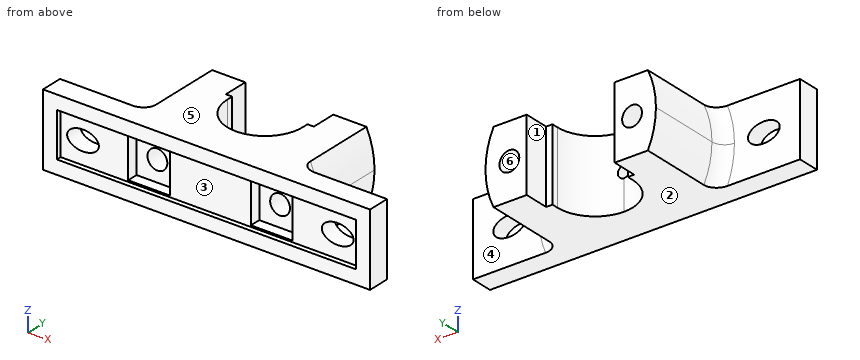
from build123d import *

# Parameters (mm, degrees)
BOSS_EXTRUDE1_DEPTH = 18.25
CUT_EXTRUDE1_START  = -43
CUT_EXTRUDE1_DEPTH  = 48
SKETCH6_R           = 5
CUT_EXTRUDE3_DEPTH  = 54.1
SKETCH7_RX          = 8
SKETCH7_RY          = 5
CUT_EXTRUDE4_DEPTH  = 11.1
FILLET3_R           = 6.4
SKETCH10_W          = 151
SKETCH10_H          = 22.5
CUT_EXTRUDE7_DEPTH  = 2.5
SKETCH11_W          = 21
SKETCH11_H          = 21
CUT_EXTRUDE8_DEPTH  = 8


with BuildPart() as part:
    # Sketch2 → Boss-Extrude1 (new, symmetric)
    with BuildSketch(Plane.XY):
        with BuildLine():
            Line((0, 0), (0, 11.1))
            Line((0, 11.1), (39.5, 11.1))
            Line((39.5, 11.1), (39.5, 54.1))
            Line((39.5, 54.1), (60.3, 54.1))
            Line((60.3, 54.1), (60.3, 41.4))
            Line((60.3, 41.4), (63.5, 41.4))
            Line((63.5, 41.4), (63.5, 38.2))
            ThreePointArc((63.5, 38.2), (69.064971157, 24.764971157), (82.5, 19.2))
            Line((82.5, 19.2), (82.5, 0))
            Line((82.5, 0), (0, 0))
        make_face()
    extrude(amount=BOSS_EXTRUDE1_DEPTH, both=True)

    # Sketch3 → Cut-Extrude1 (cut)
    with BuildSketch(Plane(origin=(0, 54.1, 0), x_dir=(1, 0, 0), z_dir=(0, 1, 0)).offset(CUT_EXTRUDE1_START)):
        with BuildLine():
            Line((39.5, -18.25), (43.564957943, -18.25))
            ThreePointArc((43.564957943, -18.25), (40.528540599, -9.348614644), (39.5, 0))
            Line((39.5, 0), (39.5, -18.25))
        make_face()
    cut_extrude1 = extrude(amount=CUT_EXTRUDE1_DEPTH, mode=Mode.SUBTRACT)

    # Mirror2: Cut-Extrude1 across plane
    add(cut_extrude1.mirror(Plane.XY), mode=Mode.SUBTRACT)

    # Mirror3: part across plane


with BuildPart() as part_1:
    add(part.part)
    add(part.part.mirror(Plane(origin=(82.5, 19.2, 18.25), x_dir=(0, 0, 1), z_dir=(1, 0, 0))))

    # Sketch6 → Cut-Extrude3 (cut)
    with BuildSketch(Plane(origin=(0, 54.1, 0), x_dir=(1, 0, 0), z_dir=(0, 1, 0))):
        with Locations(Location((51.55, 0, 0), (0, 0, 270))):
            Circle(SKETCH6_R)
    cut_extrude3 = extrude(amount=-CUT_EXTRUDE3_DEPTH, mode=Mode.SUBTRACT)

    # Sketch7 → Cut-Extrude4 (cut)
    with BuildSketch(Plane(origin=(0, 11.1, 0), x_dir=(1, 0, 0), z_dir=(0, 1, 0))):
        with Locations((18.25, 0)):
            Ellipse(SKETCH7_RX, SKETCH7_RY)
    cut_extrude4 = extrude(amount=-CUT_EXTRUDE4_DEPTH, mode=Mode.SUBTRACT)

    # Mirror4: Cut-Extrude3, Cut-Extrude4 across plane
    add(cut_extrude3.mirror(Plane.ZY.offset(-82.5)), mode=Mode.SUBTRACT)
    add(cut_extrude4.mirror(Plane.ZY.offset(-82.5)), mode=Mode.SUBTRACT)

    # Fillet3
    fillet3_edges = [part_1.edges().sort_by_distance(p)[0] for p in [
        (39.5, 11.1, 0),
        (125.5, 11.1, 0),
    ]]
    fillet(fillet3_edges, radius=FILLET3_R)

    # Sketch10 → Cut-Extrude7 (cut)
    with BuildSketch(Plane.XZ):
        with Locations((82.5, 0)):
            Rectangle(SKETCH10_W, SKETCH10_H)
    extrude(amount=-CUT_EXTRUDE7_DEPTH, mode=Mode.SUBTRACT)

    # Sketch11 → Cut-Extrude8 (cut)
    with BuildSketch(Plane.XZ):
        with Locations((51.55, 0)):
            Rectangle(SKETCH11_W, SKETCH11_H)
    cut_extrude8 = extrude(amount=-CUT_EXTRUDE8_DEPTH, mode=Mode.SUBTRACT)

    # Mirror5: Cut-Extrude8 across plane
    add(cut_extrude8.mirror(Plane.ZY.offset(-82.5)), mode=Mode.SUBTRACT)

    # Sketch12 → Cut-Revolve1 (revolve, cut)
    with BuildSketch(Plane.ZY.offset(-82.5)):
        Polygon((0, 19.5), (3, 19.5), (3, 13.5), (0, 9.983740964), align=None)
    revolve(axis=Axis((82.5, 59.1, 0), (0, -1, 0)), mode=Mode.SUBTRACT)


solid = part_1.part
CAD build for the part. Positions are in the model's coordinates, mm. Face numbers are marked on the shaded views. A direction names the side the tool comes from. Round coordinates to 2 decimals unless told otherwise and drop trailing zeros. Write each loop counter-clockwise with the first axis right and the second up, starting at its lowest first coordinate (ties: lowest second). Pieces come first, ordered by that corner, then holes.
(1) Slice it at A-A, the plane y = 47. Write the cut outline in (x, z).
(2) 3-axis set-ups, long thin cutter, end or side, ignore diameter. For the marked faces 1, 2 and 3: which of +Z, -Z, +X, -X, +Y, -Y reach the whole face in a straight line?
(3) Slice it at D-D, the plane y = 15. Write the cut outline in (x, z), and give its area (4 significant figures).
(4) Mould opens along Z. For the marked faces 4, 5 and 6 say: pulls with the +Z half, pulls with the -Z half, needs draft (parallel to the pull), parting line crosses it, or undercut.
(5) Drop flat-ended pins along their axis: P1, Ø3.5, axis at y = 39, z = 1, coming from the +X side; P2, Ø7, axis at x = 82.5, z = 0, coming from the +Y side; P3, Ø10, axis at y = 51, z = 8, coming from the +X side; P4, Ø3, axis at x = 22.5, z = -1, coming from the -Y side. Give the stop position or say it passes through.
(6) Probe line 1 along X through (y, z) = (43, 0); line 2 along Z through (x, y) = (18, 8); line 3 along X through (y, z) = (27, 0). List the from-to ranges inside material, lowest first.
(7) Slice it at B-B, the plane x = 51.55. Write the cut outline in (y, z).
(8) Slice it at C-C, the plane y = 33.5. Write the cut outline in (x, z), and give its area (3 significant figures).
From the geometry:
1. outline: (43.56, -18.25) - (60.3, -18.25) - (60.3, 18.25) - (43.56, 18.25) arc R43 ccw to start; (104.7, -18.25) - (121.44, -18.25) arc R43 ccw to (121.44, 18.25) - (104.7, 18.25) - close; hole circle Ø10 at (51.55, 0); hole circle Ø10 at (113.45, 0)
2. face 1: +Z, -Z, +Y
2. face 2: -Z, +X, -X, +Y, -Y
2. face 3: -Y
3. outline: (43, -18.25) - (122, -18.25) arc R43.51 ccw to (122, 18.25) - (43, 18.25) arc R43.51 ccw to start; hole circle Ø10 at (51.55, 0); hole circle Ø6 at (82.5, 0); hole circle Ø10 at (113.45, 0)
3. area: 2,895 mm2
4. face 4: needs draft
4. face 5: pulls with the +Z half
4. face 6: undercut
5. P1: stops at x = 125.5
5. P2: stops at y = 19.53
5. P3: stops at x = 125.4
5. P4: passes through
6. line 1: x = 39.5 to 46.55, 56.55 to 60.3, 104.7 to 108.45, 118.45 to 125.5
6. line 2: z = -18.25 to -5, 5 to 18.25
6. line 3: x = 39.5 to 46.55, 56.55 to 67.15, 97.85 to 108.45, 118.45 to 125.5
7. outline: (0, -18.25) - (54.1, -18.25) - (54.1, -5) - (8, -5) - (8, -10.5) - (2.5, -10.5) - (2.5, -11.25) - (0, -11.25) - close; (0, 11.25) - (2.5, 11.25) - (2.5, 10.5) - (8, 10.5) - (8, 5) - (54.1, 5) - (54.1, 18.25) - (0, 18.25) - close
8. outline: (43.56, -18.25) - (64.09, -18.25) - (64.09, 18.25) - (43.56, 18.25) arc R43 ccw to start; (100.91, -18.25) - (121.44, -18.25) arc R43 ccw to (121.44, 18.25) - (100.91, 18.25) - close; hole circle Ø10 at (51.55, 0); hole circle Ø10 at (113.45, 0)
8. area: 1,540 mm2
